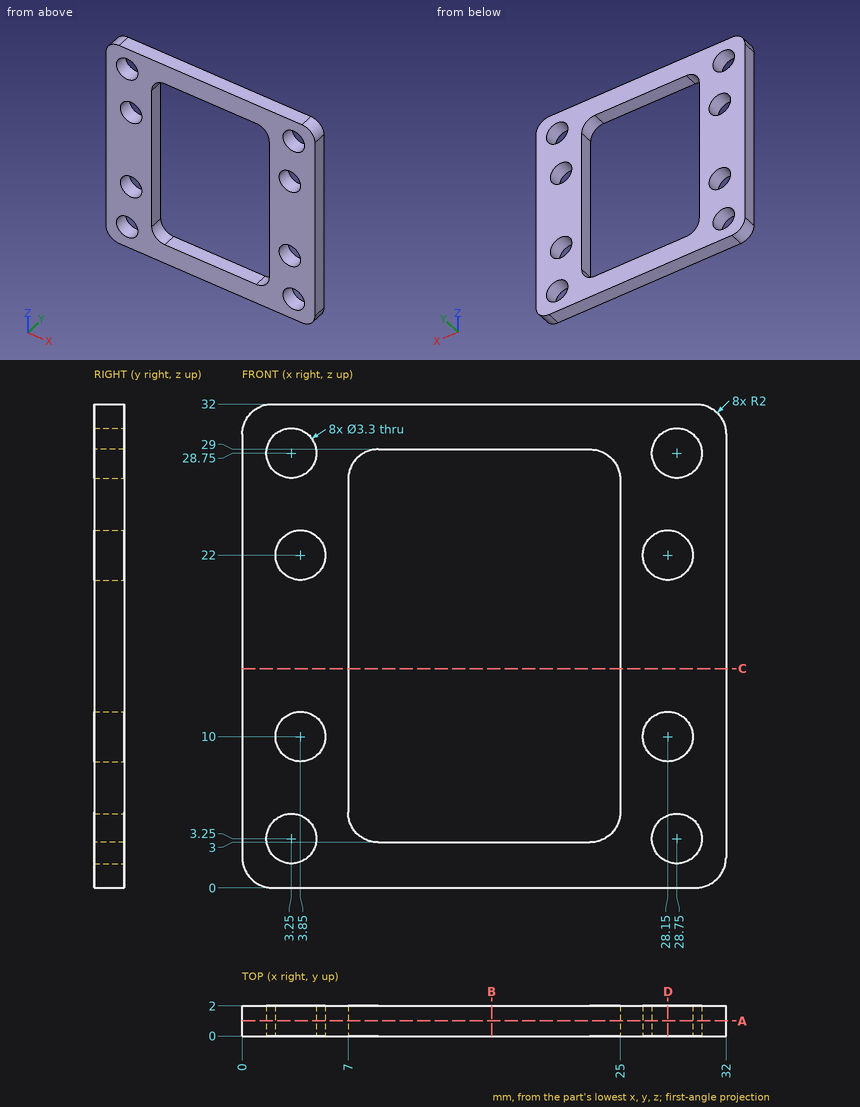
Drawing for the job (mm, zero at the part's lowest x, y, z). Give positions to 0.01 mm unless a question says otherwise; leave off trailing zeros. Order: outer loops, then holes, each group sorted by start corner. A loop starts at its lowest first (then second) coordinate and runs counter-clockwise, first axis right, second up. Notation, with made-up numbers: (61, -29) - (94, -29) arc R12 cw to (94, -6) - close; hole circle Ø1 at (0, -24). An arc over 180 degrees is marked (long way). Write item = value, one per line. Start each with the question number.
1. Cut at D-D, the plane x = 28.15. List the corners of the cut face in (y, z).
2. Cut at B-B, the plane x = 16.5. List the corners of the cut face in (y, z).
3. Cut at C-C, the plane z = 14.5. List the corners of the cut face in (x, y), and give its area (3 significant figures).
4. Cut at A-A, the plane y = 1. State how many separate pieces and enclosed holes the cut face has, and give its area (3 significant figures).
5. Probe line 1 along X through (y, z) = (1.4, 10); line 2 along X through (y, z) = (1.1, 2); line 3 along X through (y, z) = (0.4, 14). List the from-to ranges inside material, lowest first.
Taken from the geometry:
q1.outline = (0, 0) - (2, 0) - (2, 1.71) - (0, 1.71) - close; (0, 4.79) - (2, 4.79) - (2, 8.35) - (0, 8.35) - close; (0, 11.65) - (2, 11.65) - (2, 20.35) - (0, 20.35) - close; (0, 23.65) - (2, 23.65) - (2, 27.21) - (0, 27.21) - close; (0, 30.29) - (2, 30.29) - (2, 32) - (0, 32) - close
q2.outline = (0, 0) - (2, 0) - (2, 3) - (0, 3) - close; (0, 29) - (2, 29) - (2, 32) - (0, 32) - close
q3.outline = (0, 0) - (7, 0) - (7, 2) - (0, 2) - close; (25, 0) - (32, 0) - (32, 2) - (25, 2) - close
q3.area = 28.0 mm²
q4.separate_pieces = 1
q4.enclosed_holes = 9
q4.area = 488 mm²
q5.line_1 = 0 to 2.2, 5.5 to 7, 25 to 26.5, 29.8 to 32
q5.line_2 = 0 to 2.17, 4.33 to 27.67, 29.83 to 32
q5.line_3 = 0 to 7, 25 to 32
